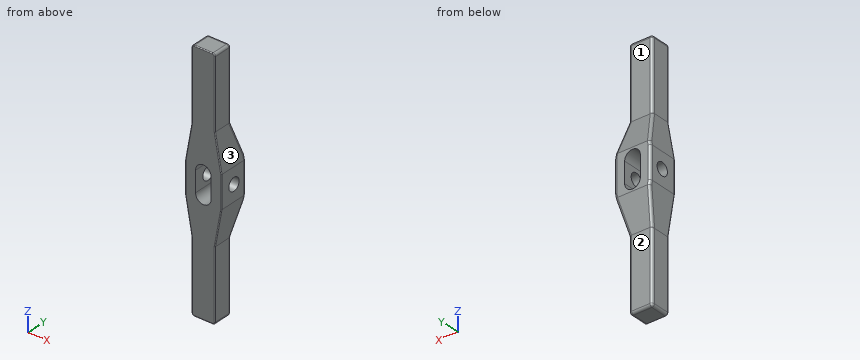
```python
from build123d import *

# Parameters (mm, degrees)
EXTRUDE1_DEPTH     = 18.415
CUT_EXTRUDE1_DEPTH = 23.225
SKETCH3_R          = 3.95605
CUT_EXTRUDE2_DEPTH = 23.225
FILLET1_R          = 1.524
FILLET2_R          = 0.508
FILLET3_R          = 1.524


with BuildPart() as part:
    # Sketch1 → Extrude1 (new body)
    with BuildSketch(Plane(origin=(0, 0, 0), x_dir=(1, 0, 0), z_dir=(0, 1, 0))):
        Polygon((-7.1374, 76.2), (7.1374, 76.2), (7.1374, 32.258), (11.1125, 9.902952), (11.1125, -9.902952), (7.1374, -32.258), (7.1374, -76.2), (-7.1374, -76.2), (-7.1374, -32.258), (-11.1125, -9.902952), (-11.1125, 9.902952), (-7.1374, 32.258), align=None)
        with BuildLine():
            Line((-4.8133, 6.35), (-4.8133, -6.35))
            ThreePointArc((-4.8133, -6.35), (0, -11.1633), (4.8133, -6.35))
            Line((4.8133, -6.35), (4.8133, 6.35))
            ThreePointArc((4.8133, 6.35), (0, 11.1633), (-4.8133, 6.35))
        make_face(mode=Mode.SUBTRACT)
    extrude(amount=EXTRUDE1_DEPTH)

    # Sketch2 → Cut-Extrude1 (cut, through all)
    with BuildSketch(Plane(origin=(11.1125, 0, 0), x_dir=(0, 0, -1), z_dir=(1, 0, 0))):
        Polygon((76.2, 18.415), (12.3698, 18.415), (31.913090461, 12.065), (76.2, 12.065), align=None)
        Polygon((-76.2, 12.065), (-76.2, 18.415), (-12.3698, 18.415), (-31.913090461, 12.065), align=None)
    extrude(amount=-CUT_EXTRUDE1_DEPTH, mode=Mode.SUBTRACT)

    # Sketch3 → Cut-Extrude2 (cut, through all)
    with BuildSketch(Plane(origin=(11.1125, 0, 0), x_dir=(0, 0, -1), z_dir=(1, 0, 0))):
        with Locations((0, 9.525)):
            Circle(SKETCH3_R)
    extrude(amount=-CUT_EXTRUDE2_DEPTH, mode=Mode.SUBTRACT)

    # Fillet1
    fillet1_edges = [part.edges().sort_by_distance(p)[0] for p in [
        (-7.1374, 6.0325, -76.2),
        (7.1374, 6.0325, -76.2),
        (7.1374, 6.0325, 76.2),
        (-7.1374, 6.0325, 76.2),
    ]]
    fillet(fillet1_edges, radius=FILLET1_R)

    # Fillet2
    fillet2_edges = [part.edges().sort_by_distance(p)[0] for p in [
        (-7.1374, 0, -53.467),
        (7.1374, 0, 53.467),
        (0, 0, 76.2),
        (0, 0, -76.2),
        (-6.691030735, 0, 75.753630735),
        (9.12495, 0, -21.080476),
        (6.691030735, 0, 75.753630735),
        (6.691030735, 0, -75.753630735),
        (-6.691030735, 0, -75.753630735),
        (11.1125, 0, 0),
        (9.12495, 0, 21.080476),
        (-7.1374, 0, 53.467),
        (-9.12495, 0, 21.080476),
        (-11.1125, 0, 0),
        (-9.12495, 0, -21.080476),
        (7.1374, 0, -53.467),
    ]]
    fillet(fillet2_edges, radius=FILLET2_R)

    # Fillet3
    fillet3_edges = [part.edges().sort_by_distance(p)[0] for p in [
        (0, 12.065, -76.2),
        (7.1374, 12.065, -53.467),
        (6.691030735, 12.065, -75.753630735),
        (-6.691030735, 12.065, -75.753630735),
        (0, 12.065, 76.2),
        (-7.1374, 12.065, 53.467),
        (-6.691030735, 12.065, 75.753630735),
        (6.691030735, 12.065, 75.753630735),
        (-11.1125, 18.415, 0),
        (-10.893176662, 18.415, 11.136376),
        (11.1125, 18.415, 0),
        (10.893176662, 18.415, -11.136376),
        (8.936291994, 15.24, -22.141445231),
        (7.168065331, 12.065, -32.085545231),
        (-10.893176662, 18.415, -11.136376),
        (-7.168065331, 12.065, -32.085545231),
        (-7.1374, 12.065, -53.467),
        (-8.936291994, 15.24, -22.141445231),
        (10.893176662, 18.415, 11.136376),
        (8.936291994, 15.24, 22.141445231),
        (7.168065331, 12.065, 32.085545231),
        (-7.168065331, 12.065, 32.085545231),
        (7.1374, 12.065, 53.467),
        (-8.936291994, 15.24, 22.141445231),
    ]]
    fillet(fillet3_edges, radius=FILLET3_R)


solid = part.part
```
For this review, take the finished solid that the model builds, in its own axes (mm). Face numbers are marked on the shaded views. A direction names the side the tool comes from. Round coordinates to 2 decimals unless told otherwise and drop trailing zeros. Write each loop counter-clockwise with the first axis right and the second up, starting at its lowest first coordinate (ties: lowest second). Pieces come first, ordered by that corner, then holes. Notation, with made-up numbers: (23.25, 54) -> (79.25, 54) arc R27 cw to (79.25, 84) -> close; hole circle Ø8 at (71, 3). An arc over 180 degrees is marked (long way). Use one line per item in the form item = value.
1) Take a section at C-C, the plane y = 4.25. Write out the cut boundary in (x, z).
Found:
outline = (-11.11, -9.9) -> (-7.14, -32.26) -> (-7.14, -74.68) arc R1.52 ccw to (-5.61, -76.2) -> (5.61, -76.2) arc R1.52 ccw to (7.14, -74.68) -> (7.14, -32.26) -> (11.11, -9.9) -> (11.11, 9.9) -> (7.14, 32.26) -> (7.14, 74.68) arc R1.52 ccw to (5.61, 76.2) -> (-5.61, 76.2) arc R1.52 ccw to (-7.14, 74.68) -> (-7.14, 32.26) -> (-11.11, 9.9) -> close; hole (-4.81, -6.35) arc R4.81 ccw to (4.81, -6.35) -> (4.81, 6.35) arc R4.81 ccw to (-4.81, 6.35) -> close
2) Take a section at B-B, the plane x = 0. Write out the cut boundary in (y, z) (3 decimals), and give its area (3 significant figures).
Found:
outline = (0, -75.692) arc R0.508 ccw to (0.508, -76.2) -> (10.541, -76.2) arc R1.524 ccw to (12.065, -74.676) -> (12.065, -31.913) -> (18.415, -12.37) -> (18.415, -11.163) -> (0, -11.163) -> close; (0, 11.163) -> (18.415, 11.163) -> (18.415, 12.37) -> (12.065, 31.913) -> (12.065, 74.676) arc R1.524 ccw to (10.541, 76.2) -> (0.508, 76.2) arc R0.508 ccw to (0, 75.692) -> close
area = 1,710 mm2
3) Clearance check with flat-ended pins moving along their axes: pin 1 (3 mm diameter, centred on y = 7.5, z = -62, fed in from -X); pin 2 (12.5 mm diameter, centred on x = -0.5, z = 59, fed in from +Y) (3 decimals); pin 3 (6 mm diameter, centred on y = 11, z = 16.5, fed in from -X). State where each tip first meets the part, or that it passes through.
Found:
pin_1 = -7.14
pin_2 = 12.065
pin_3 = -10.47
4) To check wall thickness, follow L1, parallel to Y at x = 7.5, z = 0 (3 decimals); L2, parallel to X at y = 10, z = -39.5; L3, parallel to Y at x = 3.25, z = 35 (3 decimals). State the ranges of each line that lie inside material, in increasing order. Write a range as from..to.
Found:
L1 = 0..5.569, 13.481..18.415
L2 = -7.14..7.14
L3 = 0..12.065
5) Take a section at A-A, the plane z = 0. Write out the cut boundary in (x, y) (1 decimal), and give its area (3 significant figures).
Found:
outline = (-11.1, 0.5) arc R0.5 ccw to (-10.6, 0) -> (-4.8, 0) -> (-4.8, 5.6) -> (-11.1, 5.6) -> close; (-11.1, 13.5) -> (-4.8, 13.5) -> (-4.8, 18.4) -> (-9.6, 18.4) arc R1.5 ccw to (-11.1, 16.9) -> close; (4.8, 0) -> (10.6, 0) arc R0.5 ccw to (11.1, 0.5) -> (11.1, 5.6) -> (4.8, 5.6) -> close; (4.8, 13.5) -> (11.1, 13.5) -> (11.1, 16.9) arc R1.5 ccw to (9.6, 18.4) -> (4.8, 18.4) -> close
area = 131 mm2
6) Take a section at D-D, the plane z = 59. Write out the cut boundary in (x, y) (3 decimals), and give its area (3 significant figures).
Found:
outline = (-7.137, 0.508) arc R0.508 ccw to (-6.629, 0) -> (6.629, 0) arc R0.508 ccw to (7.137, 0.508) -> (7.137, 10.541) arc R1.524 ccw to (5.613, 12.065) -> (-5.613, 12.065) arc R1.524 ccw to (-7.137, 10.541) -> close
area = 171 mm2
7) Tool access review of the marked faces 1, 2 and 3: name each direction out of +Z, -Z, +X, -X, +Y, -Y from which nothing blocks a thin tool from reaching the whole face with its end or side.
Found:
face_1 = +Z, +X, -X, +Y
face_2 = -Z, +X, -X, +Y
face_3 = +Z, +X, +Y, -Y
